Here's the drawing with two shaded views (mm, measured from the low corner). I have some questions. A direction names the side the tool comes from. Coordinates: 2 decimals unless noted, no trailing zeros. Loops run counter-clockwise (first coordinate to the right, second up) from the corner with the lowest first, then second, coordinate; pieces in that order, holes last. Notation, with made-up numbers: (89, 31.25) -> (141, 31.25) arc R22 cw to (141, 67.25) -> close; hole circle Ø6 at (-32, 65). An arc over 180 degrees is marked (long way). Answer as a JSON object with one key per item and string values. Group by question number.
Q1. I want a section at D-D on z = 15. Write out the boundary of the cut face in (x, y).
Q2. On a 3-axis mill with a long thin cutter (end or side, diameter ignored), from which of +Z, -Z, +X, -X, +Y, -Y can I reach the whole of each face in a straight line? I mean the marked faces 1 and 2. Say none if no direction works.
Q3. I need wall thicknesses on line 1 (Z direction, x = 11, y = 16.5); line 2 (X direction, y = 11, z = 4); line 3 (X direction, y = 4.75, z = 2.75). Which ranges of each line are inside material? Lowest first, please.
Q4. Thinking about a two-plate mould opening in X: for the marked faces 3 and 4, which applies, released by +X, released by -X, zero draft, split by the parting line, or undercut?
Q5. I'm going to push flat-ended pins straight in: pin 1 (8 mm diameter, centred on y = 8.5, z = 17.5, fed in from -X); pin 2 (6 mm diameter, centred on y = 7, z = 21.5, fed in from +X); pin 3 (8 mm diameter, centred on y = 2.5, z = 18, fed in from -X). Where does each tip first touch, or does it pass through?
Q6. I want a section at C-C on z = 6. Write out the boundary of the cut face in (x, y), then the cut area to 3 significant figures.
Q7. I want a section at A-A on y = 10. Write out the boundary of the cut face in (x, z), then the cut area to 3 significant figures.
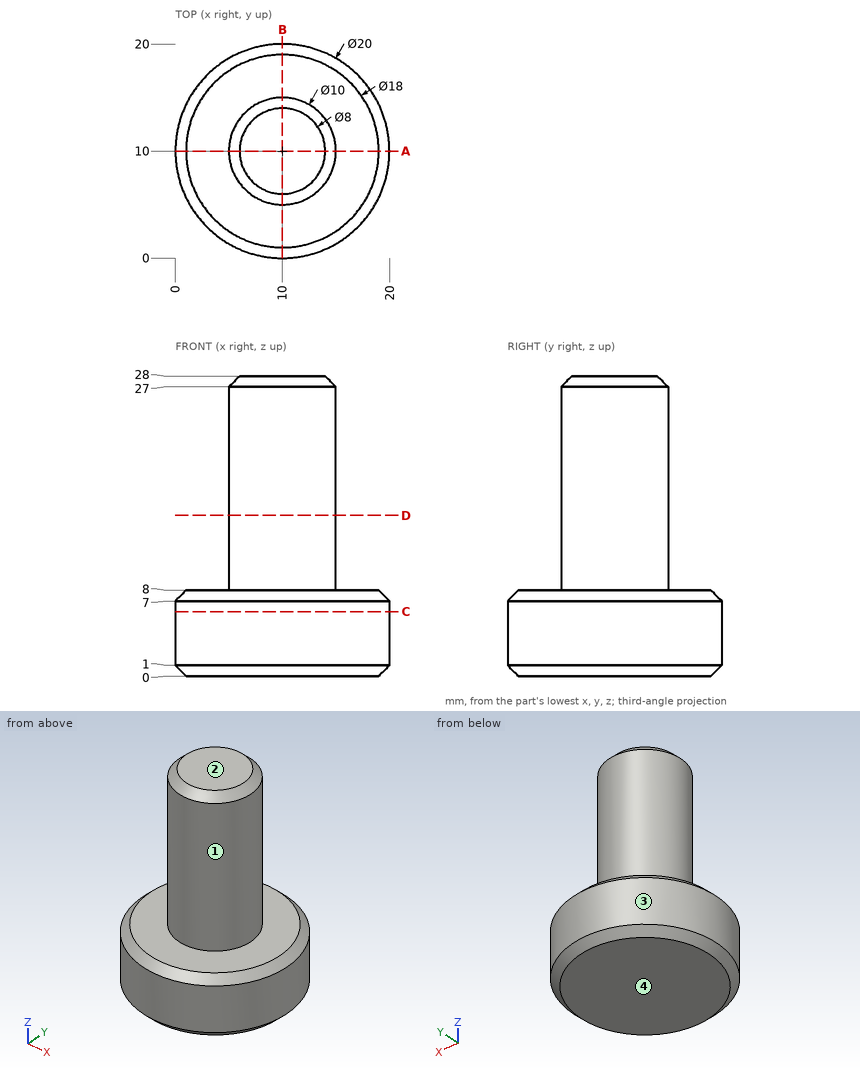
Result set:
{
 "1": {"outline": "circle Ø10 at (10, 10)"},
 "2": {"face 1": "+Z", "face 2": "+Z, +X, -X, +Y, -Y"},
 "3": {"line 1": "z = 0 to 8", "line 2": "x = 0.05 to 19.95", "line 3": "x = 1.49 to 18.51"},
 "4": {"face 3": "split by the parting line", "face 4": "zero draft"},
 "5": {"pin 1": "stops at x = 5", "pin 2": "stops at x = 15", "pin 3": "stops at x = 6.43"},
 "6": {"outline": "circle Ø20 at (10, 10)", "area": "314 mm²"},
 "7": {"outline": "(0, 1) -> (1, 0) -> (19, 0) -> (20, 1) -> (20, 7) -> (19, 8) -> (15, 8) -> (15, 27) -> (14, 28) -> (6, 28) -> (5, 27) -> (5, 8) -> (1, 8) -> (0, 7) -> close", "area": "357 mm²"}
}
